```python
from build123d import *

# Parameters (mm, degrees)
SKETCH1_W           = 4
SKETCH1_H           = 15.2
BOSS_EXTRUDE1_DEPTH = 1
SKETCH2_W           = 4
SKETCH2_H           = 4.9
BOSS_EXTRUDE2_DEPTH = 4
CUT_EXTRUDE2_REACH  = 18.126
SKETCH4_R           = 0.75


with BuildPart() as part:
    # Sketch1 → Boss-Extrude1 (new body)
    with BuildSketch(Plane(origin=(0, 0, 0), x_dir=(1, 0, 0), z_dir=(0, 1, 0))):
        Rectangle(SKETCH1_W, SKETCH1_H)
    extrude(amount=BOSS_EXTRUDE1_DEPTH)

    # Sketch2 → Boss-Extrude2 (add)
    with BuildSketch(Plane(origin=(0, 1, 0), x_dir=(1, 0, 0), z_dir=(0, 1, 0))):
        with Locations((0, -5.15)):
            Rectangle(SKETCH2_W, SKETCH2_H)
    boss_extrude2 = extrude(amount=BOSS_EXTRUDE2_DEPTH)

    # Sketch4 → Cut-Extrude2 (cut, up to next)
    with BuildSketch(Plane.XY.offset(7.6), mode=Mode.PRIVATE) as cut_extrude2_sk1:
        with Locations((0.5, 2.5)):
            Circle(SKETCH4_R)
    cut_extrude2_tool1 = extrude(cut_extrude2_sk1.sketch, amount=-CUT_EXTRUDE2_REACH, mode=Mode.PRIVATE) & part.part
    cut_extrude2 = cut_extrude2_tool1.solids().sort_by_distance((0.5, 2.5, 7.6))[0]
    add(cut_extrude2, mode=Mode.SUBTRACT)

    # Mirror3: Boss-Extrude2, Cut-Extrude2 across plane
    add(boss_extrude2.mirror(Plane.XY))
    add(cut_extrude2.mirror(Plane.XY), mode=Mode.SUBTRACT)


solid = part.part
```
The model under review builds one solid part; all positions refer to its coordinate system, in mm. A direction names the side the tool comes from. Give positions to 0.01 mm unless a question says otherwise; leave off trailing zeros. Write each loop counter-clockwise with the first axis right and the second up, starting at its lowest first coordinate (ties: lowest second). Pieces come first, ordered by that corner, then holes. Notation, with made-up numbers: (60.25, -27) - (84.25, -27) arc R15 cw to (84.25, -16) - close; hole circle Ø1 at (-33.75, 30). An arc over 180 degrees is marked (long way). Answer in a Markdown table with one row per item. Add a question column.
1. We need section C-C on y = 4.4. Write out the cut boundary in (x, z), then the cut area to 3 significant figures.
2. We need section B-B on x = 0.5. Write out the cut boundary in (y, z).
3. Tool access review of faces 1 (the flat face through (-2, 0.8, -0.1)), 2 (the flat face through (-0.5, 3, -2.7)): name each direction out of +Z, -Z, +X, -X, +Y, -Y from which nothing blocks a thin tool from reaching the whole face with its end or side.
4. Wall thickness on line 1 along Z through (x, y) = (-1.15, 2.5); line 2 along Y through (x, z) = (0.5, 4.15); line 3 along Y through (x, z) = (-0.3, 2.5): over which ranges is each line inside the solid? List them lowest first. Write a range as [from, to].
5. We need section D-D on z = 6.25. Write out the cut boundary in (x, y).
6. Draft analysis for pull direction Z (two halves, no side actions). For faces 3 (the flat face through (-0.5, 2.5, 7.6)), 4 (the flat face through (0, 5, -5)), 5 (the flat face through (-0.5, 3, 2.7)), state which applies: +Z half, -Z half, draft (parallel to the pull), parting line (faces both ways), or undercut.
7. We need section A-A on y = 2.5. Write out the cut boundary in (x, z).
8. Insertion check: P1, Ø1, axis at x = -0.5, z = 0, coming from the +Y side; P2, Ø1.2, axis at x = 0.5, y = 2.5, coming from the -Z side. Each pin has a flat end and moves straight along its axis. Give the tip position at first contact, or say it passes through.
Ans:
| question | item | result |
|---|---|---|
| 1 | outline | (-2, -7.6) - (2, -7.6) - (2, -2.7) - (-2, -2.7) - close; (-2, 2.7) - (2, 2.7) - (2, 7.6) - (-2, 7.6) - close |
| 1 | area | 39.2 mm^2 |
| 2 | outline | (0, -7.6) - (1.75, -7.6) - (1.75, -2.7) - (1, -2.7) - (1, 2.7) - (1.75, 2.7) - (1.75, 7.6) - (0, 7.6) - close; (3.25, -7.6) - (5, -7.6) - (5, -2.7) - (3.25, -2.7) - close; (3.25, 2.7) - (5, 2.7) - (5, 7.6) - (3.25, 7.6) - close |
| 3 | face 1 | +Z, -Z, -X, +Y, -Y |
| 3 | face 2 | +X, -X, +Y |
| 4 | line 1 | z = [-7.6, -2.7], [2.7, 7.6] |
| 4 | line 2 | y = [0, 1.75], [3.25, 5] |
| 4 | line 3 | y = [0, 1] |
| 5 | outline | (-2, 0) - (2, 0) - (2, 5) - (-2, 5) - close; hole circle Ø1.5 at (0.5, 2.5) |
| 6 | face 3 | +Z half |
| 6 | face 4 | draft |
| 6 | face 5 | undercut |
| 7 | outline | (-2, -7.6) - (-0.25, -7.6) - (-0.25, -2.7) - (-2, -2.7) - close; (-2, 2.7) - (-0.25, 2.7) - (-0.25, 7.6) - (-2, 7.6) - close; (1.25, -7.6) - (2, -7.6) - (2, -2.7) - (1.25, -2.7) - close; (1.25, 2.7) - (2, 2.7) - (2, 7.6) - (1.25, 7.6) - close |
| 8 | P1 | stops at y = 1 |
| 8 | P2 | passes through |
